from build123d import *

# Parameters (mm, degrees)
BOSS_EXTRUDE1_DEPTH      = 200
BOSS_EXTRUDE1_DEPTH_BACK = 150
SKETCH1_W                = 50
SKETCH1_H                = 2
SKETCH2_R                = 11
CUT_EXTRUDE1_DEPTH       = 202.566366242


with BuildPart() as part:
    # Sketch1 → Boss-Extrude1 (new, two sides: drawn at the far end of the back side and taken through both)
    with BuildSketch(Plane(origin=(0, 0, 0), x_dir=(1, 0, 0), z_dir=(0, 1, 0)).offset(-BOSS_EXTRUDE1_DEPTH_BACK)):
        Rectangle(SKETCH1_W, SKETCH1_H)
    extrude(amount=BOSS_EXTRUDE1_DEPTH + BOSS_EXTRUDE1_DEPTH_BACK)

    # Sketch2 → Cut-Extrude1 (cut, through all)
    with BuildSketch(Plane(origin=(0, 0, -1), x_dir=(-1, 0, 0), z_dir=(0, 0, -1))):
        with Locations((-4, -109)):
            Circle(SKETCH2_R)
    extrude(amount=-CUT_EXTRUDE1_DEPTH, mode=Mode.SUBTRACT)


solid = part.part
Source: CAD feature listing. Evaluate the final solid. Frame: model axes, mm. Give positions to 0.01 mm unless a question says otherwise; leave off trailing zeros. Write each loop counter-clockwise with the first axis right and the second up, starting at its lowest first coordinate (ties: lowest second). Pieces come first, ordered by that corner, then holes. Notation, with made-up numbers: (69.5, -27) -> (99.5, -27) arc R14 ccw to (99.5, -15) -> close; hole circle Ø2 at (51.5, 28). An arc over 180 degrees is marked (long way). Return JSON: item names as keys, results as strings. Group by question number.
1. Section C-C, the plane z = 0.25. Output: boundary loops of the cut face in (x, y), then the cut area to 3 significant figures.
2. Material intervals for line 1 (Y direction, x = 4, z = 0.25); line 2 (Y direction, x = 10.5, z = 0.25); line 3 (X direction, y = -99, z = -0.65), sorted ascending. Write a range as from..to.
3. Section B-B, the plane x = 4. Output: boundary loops of the cut face in (y, z).
4. Section A-A, the plane y = -109. Output: boundary loops of the cut face in (x, z), then the cut area to 3 significant figures.
5. Mould query, pull axis Y, two halves, no side actions, for faces 1 (the face through (0, 23, -1)), 2 (the face through (5.432, -98.094, -0.014)). Classes: +Y half, -Y half, draft (parallel to the pull), parting line (faces both ways), or undercut.
Determined:
{
 "1": {"outline": "(-25, -150) -> (25, -150) -> (25, 200) -> (-25, 200) -> close; hole circle Ø22 at (4, -109)", "area": "17,100 mm2"},
 "2": {"line 1": "y = -150..-120, -98..200", "line 2": "y = -150..-117.87, -100.13..200", "line 3": "x = -25..-0.58, 8.58..25"},
 "3": {"outline": "(-150, -1) -> (-120, -1) -> (-120, 1) -> (-150, 1) -> close; (-98, -1) -> (200, -1) -> (200, 1) -> (-98, 1) -> close"},
 "4": {"outline": "(-25, -1) -> (-7, -1) -> (-7, 1) -> (-25, 1) -> close; (15, -1) -> (25, -1) -> (25, 1) -> (15, 1) -> close", "area": "56.0 mm2"},
 "5": {"face 1": "draft", "face 2": "undercut"}
}
